Input: part model. Units: mm. Frame: model coordinates. A direction names the side the tool comes from. Round coordinates to 2 decimals unless told otherwise and drop trailing zeros. Order: outer loops, then holes, each group sorted by start corner. A loop starts at its lowest first (then second) coordinate and runs counter-clockwise, first axis right, second up. Notation, with made-up numbers: M 88.25,28 L 96.25,28 A25 cw 96.25,41 Z; hole C -31,4 d11. An arc over 180 degrees is marked long. One line per question, with ' | ' between items.
```python
from build123d import *

# Parameters (mm, degrees)
SKETCH1_W           = 30
SKETCH1_H           = 50
BOSS_EXTRUDE1_DEPTH = 10
SKETCH2_W           = 30
SKETCH2_H           = 2
CUT_EXTRUDE3_DEPTH  = 1


with BuildPart() as part:
    # Sketch1 → Boss-Extrude1 (new body)
    with BuildSketch(Plane.XY):
        with Locations((-15, -25)):
            Rectangle(SKETCH1_W, SKETCH1_H)
    extrude(amount=BOSS_EXTRUDE1_DEPTH)

    # Sketch2 → Cut-Extrude3 (cut)
    with BuildSketch(Plane.XY.offset(10)):
        with Locations((-15, -3)):
            Rectangle(SKETCH2_W, SKETCH2_H)
        with Locations((-15, -7)):
            Rectangle(SKETCH2_W, SKETCH2_H)
        with Locations((-15, -11)):
            Rectangle(SKETCH2_W, SKETCH2_H)
        with Locations((-15, -15)):
            Rectangle(SKETCH2_W, SKETCH2_H)
        with Locations((-15, -19)):
            Rectangle(SKETCH2_W, SKETCH2_H)
        with Locations((-15, -23)):
            Rectangle(SKETCH2_W, SKETCH2_H)
        with Locations((-15, -27)):
            Rectangle(SKETCH2_W, SKETCH2_H)
        with Locations((-15, -31)):
            Rectangle(SKETCH2_W, SKETCH2_H)
        with Locations((-15, -35)):
            Rectangle(SKETCH2_W, SKETCH2_H)
        with Locations((-15, -39)):
            Rectangle(SKETCH2_W, SKETCH2_H)
        with Locations((-15, -43)):
            Rectangle(SKETCH2_W, SKETCH2_H)
        with Locations((-15, -47)):
            Rectangle(SKETCH2_W, SKETCH2_H)
    extrude(amount=-CUT_EXTRUDE3_DEPTH, mode=Mode.SUBTRACT)


solid = part.part
```
Item 1: Section query A-A, the plane y = -7.5. Return loops of the section in (x, z), plus the area to 3 significant figures.
Report:
outline: M -30,0 L 0,0 L 0,9 L -30,9 Z | area: 270 mm²
Item 2: Line query: line 1 along Z through (x, y) = (-16, -35). Output: solid intervals per line, ascending. Write a range as from..to.
Report:
line 1: 0..9
Item 3: First-contact query: pin 1 (1 mm diameter, centred on x = -22, y = -47, fed in from +Z). Flat tip, straight axial feed; report the tip coordinate or a pass-through.
Report:
pin 1: z = 9
Item 4: Access query for faces 1 (the flat face through (-15.2, -44, 9.5)), 2 (the flat face through (-15, -1, 10)). Directions: +Z, -Z, +X, -X, +Y, -Y. A direction counts if a zero-diameter tool reaches every point of the face in a straight line with its end or side. Return the directions, or none.
Report:
face 1: +Z, +X, -X | face 2: +Z, +X, -X, +Y, -Y
Item 5: Mould query, pull axis Y, two halves, no side actions, for faces 3 (the flat face through (-15, -9, 10)), 4 (the flat face through (-15, -31, 9)). Classes: +Y half, -Y half, draft (parallel to the pull), parting line (faces both ways), or undercut.
Report:
face 3: draft | face 4: undercut
